from build123d import *

# Parameters (mm, degrees)
SKETCH_1_R          = 100
SKETCH_1_R_2        = 29
EXTRUDE_1_DEPTH     = 34
SKETCH_2_R          = 85
SKETCH_2_R_2        = 44
CUT_EXTRUDE_1_DEPTH = 10


with BuildPart() as part:
    # 草图1 → 凸台-拉伸1 (new body, symmetric)
    with BuildSketch(Plane(origin=(0, 0, 0), x_dir=(1, 0, 0), z_dir=(0, 1, 0))):
        Circle(SKETCH_1_R)
        Circle(SKETCH_1_R_2, mode=Mode.SUBTRACT)
    extrude(amount=EXTRUDE_1_DEPTH, both=True)

    # 草图2 → 切除-拉伸1 (cut)
    with BuildSketch(Plane.XZ.offset(34)):
        Circle(SKETCH_2_R)
        Circle(SKETCH_2_R_2, mode=Mode.SUBTRACT)
    cut_extrude_1 = extrude(amount=-CUT_EXTRUDE_1_DEPTH, mode=Mode.SUBTRACT)

    # 镜向1: 切除-拉伸1 across plane
    add(cut_extrude_1.mirror(Plane.ZX), mode=Mode.SUBTRACT)


solid = part.part
Verification items for the finished model (mm, model axes). A direction names the side the tool comes from. Give positions to 0.01 mm unless a question says otherwise; leave off trailing zeros. Write each loop counter-clockwise with the first axis right and the second up, starting at its lowest first coordinate (ties: lowest second). Pieces come first, ordered by that corner, then holes.
(1) Cross-section at D-D (x = -65). Enter the section's corners in (y, z), plus the area to 3 significant figures.
(2) Access from +Z, -Z, +X, -X, +Y, -Y to the whole of each face (thin tool, end or side, straight path). Record for faces 5 (the face through (37, -24, -37)), 6 (the face through (13.38, -0.48, 25.73)), 7 (the face through (-9.538, 29.07, -42.954)).
(3) Cross-section at C-C (y = 4). Enter the section's corners in (x, z), plus the area to 3 significant figures.
(4) Cross-section at A-A (x = 0). Enter the section's corners in (y, z), plus the area to 3 significant figures.
(5) Mould release check, pull along Z, two halves, no side actions. Record for faces 1 (the face through (-67.453, 29.07, -51.721)), 2 (the face through (95.38, 0.48, -30.04)), 3 (the face through (-67.453, -29.07, -51.721)), 4 (the face through (29, -34, 9)): +Z half, -Z half, draft (parallel to the pull), parting line (faces both ways), or undercut.
(6) Cross-section at B-B (z = 0). Enter the section's corners in (x, y).
(7) Material ranges on line 1 (Z direction, x = 0, y = 31.25); line 2 (X direction, y = -17.5, z = 0), recorded low to high.
(8) Gauge pin test, flat ends, axial feed: pin 1 (2 mm diameter, centred on x = -40, y = -20, fed in from -Z); pin 2 (1.5 mm diameter, centred on x = -57, y = -2.5, fed in from -Z); pin 3 (1 mm diameter, centred on x = 9, y = -17, fed in from +Z). Record the tip position at first contact, or that the pin passes through.
Worked out:
1. outline: (-34, -75.99) - (34, -75.99) - (34, -54.77) - (24, -54.77) - (24, 54.77) - (34, 54.77) - (34, 75.99) - (-34, 75.99) - (-34, 54.77) - (-24, 54.77) - (-24, -54.77) - (-34, -54.77) - close
1. area: 8,140 mm2
2. face 5: -Y
2. face 6: +Y, -Y
2. face 7: +Y
3. outline: circle Ø200 at (0, 0); hole circle Ø58 at (0, 0)
3. area: 28,800 mm2
4. outline: (-34, -100) - (34, -100) - (34, -85) - (24, -85) - (24, -44) - (34, -44) - (34, -29) - (-34, -29) - (-34, -44) - (-24, -44) - (-24, -85) - (-34, -85) - close; (-34, 29) - (34, 29) - (34, 44) - (24, 44) - (24, 85) - (34, 85) - (34, 100) - (-34, 100) - (-34, 85) - (-24, 85) - (-24, 44) - (-34, 44) - close
4. area: 8,020 mm2
5. face 1: undercut
5. face 2: parting line
5. face 3: undercut
5. face 4: draft
6. outline: (-100, -34) - (-85, -34) - (-85, -24) - (-44, -24) - (-44, -34) - (-29, -34) - (-29, 34) - (-44, 34) - (-44, 24) - (-85, 24) - (-85, 34) - (-100, 34) - close; (29, -34) - (44, -34) - (44, -24) - (85, -24) - (85, -34) - (100, -34) - (100, 34) - (85, 34) - (85, 24) - (44, 24) - (44, 34) - (29, 34) - close
7. line 1: z = -100 to -85, -44 to -29, 29 to 44, 85 to 100
7. line 2: x = -100 to -29, 29 to 100
8. pin 1: stops at z = -92.08
8. pin 2: stops at z = -82.68
8. pin 3: stops at z = 99.64
